Design review of the part built by this model. Coordinates are the model's own, in mm. Face numbers are marked on the shaded views. Give positions to 0.01 mm unless a question says otherwise; leave off trailing zeros. Loops run counter-clockwise (first coordinate to the right, second up) from the corner with the lowest first, then second, coordinate; pieces in that order, holes last. Notation, with made-up numbers: M 34.5,-7.5 L 41.5,-7.5 A12 cw 41.5,5.5 Z; hole C -38.75,-8 d1. An arc over 180 degrees is marked long. Use a Markdown table: item, result. Add a question column.
(1) Insertion check: pin 1 Ø17 at (x, y) = (48.87, 80.04) entering from +Z; pin 2 Ø5 at (x, y) = (-173, -226) entering from +Z; pin 3 Ø5 at (x, y) = (-157.5, -162) entering from +Z; pin 4 Ø5.5 at (y, z) = (89, 3.5) entering from +X. Each pin has a flat end and moves straight along its axis. Give the tip position at first contact, or say it passes through.
(2) Add section D-D, the plane x = -145.5. Give the boundary of the cut face in (y, z).
(3) Add section B-B, the plane x = -110.5. Give the boundary of the cut face in (y, z).
(4) For probe 1 along Y at (x, z) = (-95, 8); probe 2 along X at (y, z) = (-222, 8); probe 3 along Y at (x, z) = (-66, 3.25), list the stretches that pass through material, from the lowest coordinate up.
(5) Add section A-A, the plane y = -22. Give the boundary of the cut face in (x, z).
(6) Add section C-C, the plane y = -169. Give the boundary of the cut face in (x, z), then the cut area to 3 significant figures.
(7) Draft analysis for pull direction X (two halves, no side actions). For the marked faces 1 and 2, state which applies: pulls with the +X half, pulls with the -X half, needs draft (parallel to the pull), parting line crosses it, or undercut.
```python
from build123d import *

# Parameters (mm, degrees)
MODEL_R                 = 10.75
MODEL_R_2               = 1.75
MODEL_R_3               = 5.25
MODEL_R_4               = 1.65
SALIENTE_EXTRUIR1_DEPTH = 10
CORTAR_EXTRUIR1_DEPTH   = 5
CORTAR_EXTRUIR2_DEPTH   = 3
CROQUIS3_R              = 5.1
CORTAR_EXTRUIR3_DEPTH   = 4
CORTAR_EXTRUIR4_REACH   = 307.225
CROQUIS4_R              = 50
CORTAR_EXTRUIR5_REACH   = 307.141


with BuildPart() as part:
    # Model → Saliente-Extruir1 (new body)
    with BuildSketch(Plane.XY):
        with BuildLine():
            Line((-155.7898, 91.0382), (-155.7898, 58.205145042))
            ThreePointArc((-155.7898, 58.205145042), (-156.112526651, 56.437911606), (-157.039045607, 54.898811501))
            Line((-157.039045607, 54.898811501), (-188.380554393, 19.344533541))
            ThreePointArc((-188.380554393, 19.344533541), (-189.307073349, 17.805433436), (-189.6298, 16.0382))
            Line((-189.6298, 16.0382), (-189.6298, -233.9618))
            ThreePointArc((-189.6298, -233.9618), (-188.165333906, -237.497333906), (-184.6298, -238.9618))
            Line((-184.6298, -238.9618), (92.3702, -238.9618))
            ThreePointArc((92.3702, -238.9618), (95.905733906, -237.497333906), (97.3702, -233.9618))
            Line((97.3702, -233.9618), (97.3702, 16.0382))
            ThreePointArc((97.3702, 16.0382), (97.047473349, 17.805433436), (96.120954393, 19.344533541))
            Line((96.120954393, 19.344533541), (64.779445607, 54.898811501))
            ThreePointArc((64.779445607, 54.898811501), (63.852926651, 56.437911606), (63.5302, 58.205145042))
            Line((63.5302, 58.205145042), (63.5302, 91.0382))
            ThreePointArc((63.5302, 91.0382), (62.065733906, 94.573733906), (58.5302, 96.0382))
            Line((58.5302, 96.0382), (-150.7898, 96.0382))
            ThreePointArc((-150.7898, 96.0382), (-154.325333906, 94.573733906), (-155.7898, 91.0382))
        make_face()
        with Locations((48.8702, 80.0382)):
            Circle(MODEL_R, mode=Mode.SUBTRACT)
        with Locations((37.5552, 68.7232)):
            Circle(MODEL_R_2, mode=Mode.SUBTRACT)
        with Locations((60.1852, 68.7232)):
            Circle(MODEL_R_2, mode=Mode.SUBTRACT)
        with Locations((60.1852, 91.3532)):
            Circle(MODEL_R_2, mode=Mode.SUBTRACT)
        with Locations((37.5552, 91.3532)):
            Circle(MODEL_R_2, mode=Mode.SUBTRACT)
        with Locations(Location((-129.8148, 91.3532, 0), (0, 0, 180))):
            Circle(MODEL_R_2, mode=Mode.SUBTRACT)
        with Locations(Location((-152.4448, 91.3532, 0), (0, 0, 180))):
            Circle(MODEL_R_2, mode=Mode.SUBTRACT)
        with Locations(Location((-152.4448, 68.7232, 0), (0, 0, 180))):
            Circle(MODEL_R_2, mode=Mode.SUBTRACT)
        with Locations(Location((-129.8148, 68.7232, 0), (0, 0, 180))):
            Circle(MODEL_R_2, mode=Mode.SUBTRACT)
        with Locations(Location((-141.1298, 80.0382, 0), (0, 0, 180))):
            Circle(MODEL_R, mode=Mode.SUBTRACT)
        with Locations((-46.1298, 80.0382)):
            Circle(MODEL_R_3, mode=Mode.SUBTRACT)
        with Locations((-51.8798, 85.7882)):
            Circle(MODEL_R_4, mode=Mode.SUBTRACT)
        with Locations((-40.3798, 85.7882)):
            Circle(MODEL_R_4, mode=Mode.SUBTRACT)
        with Locations((-40.3798, 74.2882)):
            Circle(MODEL_R_4, mode=Mode.SUBTRACT)
        with Locations((-51.8798, 74.2882)):
            Circle(MODEL_R_4, mode=Mode.SUBTRACT)
    extrude(amount=SALIENTE_EXTRUIR1_DEPTH)

    # Croquis1 → Cortar-Extruir1 (cut)
    with BuildSketch(Plane.XY.offset(10)):
        with BuildLine():
            Line((-167.1298, -229.4618), (-167.1298, 11.5382))
            ThreePointArc((-167.1298, 11.5382), (-166.983353391, 11.891753391), (-166.6298, 12.0382))
            Line((-166.6298, 12.0382), (74.3702, 12.0382))
            ThreePointArc((74.3702, 12.0382), (74.723753391, 11.891753391), (74.8702, 11.5382))
            Line((74.8702, 11.5382), (74.8702, -229.4618))
            ThreePointArc((74.8702, -229.4618), (74.723753391, -229.815353391), (74.3702, -229.9618))
            Line((74.3702, -229.9618), (-166.6298, -229.9618))
            ThreePointArc((-166.6298, -229.9618), (-166.983353391, -229.815353391), (-167.1298, -229.4618))
        make_face()
    extrude(amount=-CORTAR_EXTRUIR1_DEPTH, mode=Mode.SUBTRACT)

    # Croquis2 → Cortar-Extruir2 (cut)
    with BuildSketch(Plane.XY.offset(10)):
        with BuildLine():
            Line((-182.1298, -233.9618), (-182.1298, 16.0382))
            ThreePointArc((-182.1298, 16.0382), (-181.836906781, 16.745306781), (-181.1298, 17.0382))
            Line((-181.1298, 17.0382), (88.8702, 17.0382))
            ThreePointArc((88.8702, 17.0382), (89.577306781, 16.745306781), (89.8702, 16.0382))
            Line((89.8702, 16.0382), (89.8702, -233.9618))
            ThreePointArc((89.8702, -233.9618), (89.577306781, -234.668906781), (88.8702, -234.9618))
            Line((88.8702, -234.9618), (-181.1298, -234.9618))
            ThreePointArc((-181.1298, -234.9618), (-181.836906781, -234.668906781), (-182.1298, -233.9618))
        make_face()
    extrude(amount=-CORTAR_EXTRUIR2_DEPTH, mode=Mode.SUBTRACT)

    # Croquis3 → Cortar-Extruir3 (cut)
    with BuildSketch(Plane.XY.offset(7)):
        with Locations((-174.6298, -227.4618)):
            Circle(CROQUIS3_R)
        with Locations(Location((82.3702, -227.4618, 0), (0, 0, 180))):
            Circle(CROQUIS3_R)
        with Locations(Location((-174.6298, 9.5382, 0), (0, 0, 180))):
            Circle(CROQUIS3_R)
        with Locations((82.3702, 9.5382)):
            Circle(CROQUIS3_R)
    extrude(amount=-CORTAR_EXTRUIR3_DEPTH, mode=Mode.SUBTRACT)

    # Croquis4 → Cortar-Extruir4 (cut, up to next)
    with BuildSketch(Plane(origin=(0, 0, 0), x_dir=(-1, 0, 0), z_dir=(0, 0, -1)), mode=Mode.PRIVATE) as cortar_extruir4_sk1:
        with Locations((46.1298, -281.9618)):
            Circle(CROQUIS4_R)
    cortar_extruir4_tool1 = extrude(cortar_extruir4_sk1.sketch, amount=-CORTAR_EXTRUIR4_REACH, mode=Mode.PRIVATE) & part.part
    add(cortar_extruir4_tool1.solids().sort_by_distance((-46.1298, -281.9618, 0))[0], mode=Mode.SUBTRACT)

    # Croquis5 → Cortar-Extruir5 (cut, up to next)
    with BuildSketch(Plane.XY.offset(7), mode=Mode.PRIVATE) as cortar_extruir5_sk1:
        with BuildLine():
            Line((-71.1298, -27.9618), (-71.1298, 12.0382))
            Line((-71.1298, 12.0382), (-48.1298, 12.0382))
            Line((-48.1298, 12.0382), (-48.1298, 33.205145042))
            ThreePointArc((-48.1298, 33.205145042), (-54.866344033, 49.468601009), (-71.1298, 56.205145042))
            Line((-71.1298, 56.205145042), (-75.9598, 56.205145042))
            ThreePointArc((-75.9598, 56.205145042), (-95.051683092, 64.11326195), (-102.9598, 83.205145042))
            Line((-102.9598, 83.205145042), (-102.9598, 96.0382))
            Line((-102.9598, 96.0382), (-98.9598, 96.0382))
            Line((-98.9598, 96.0382), (-98.9598, 83.205145042))
            ThreePointArc((-98.9598, 83.205145042), (-92.223255967, 66.941689074), (-75.9598, 60.205145042))
            Line((-75.9598, 60.205145042), (-71.1298, 60.205145042))
            ThreePointArc((-71.1298, 60.205145042), (-52.037916908, 52.297028134), (-44.1298, 33.205145042))
            Line((-44.1298, 33.205145042), (-44.1298, 12.0382))
            Line((-44.1298, 12.0382), (-21.1298, 12.0382))
            Line((-21.1298, 12.0382), (-21.1298, -27.9618))
            Line((-21.1298, -27.9618), (-71.1298, -27.9618))
        make_face()
    cortar_extruir5_tool1 = extrude(cortar_extruir5_sk1.sketch, amount=-CORTAR_EXTRUIR5_REACH, mode=Mode.PRIVATE) & part.part
    add(cortar_extruir5_tool1.solids().sort_by_distance((-50.971663, 4.050415, 7))[0], mode=Mode.SUBTRACT)


solid = part.part
```
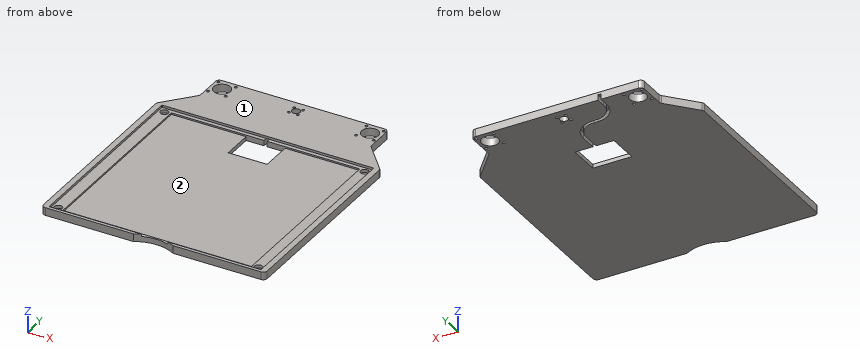
Established:
| question | item | result |
|---|---|---|
| 1 | pin 1 | through |
| 1 | pin 2 | z = 3 |
| 1 | pin 3 | z = 5 |
| 1 | pin 4 | x = 63.53 |
| 2 | outline | M -238.96,0 L 70.22,0 L 70.22,10 L 17.04,10 L 17.04,7 L 12.04,7 L 12.04,5 L -229.96,5 L -229.96,7 L -234.96,7 L -234.96,10 L -238.96,10 Z; M 89.86,0 L 96.04,0 L 96.04,10 L 89.86,10 Z |
| 3 | outline | M -238.96,0 L 96.04,0 L 96.04,10 L 17.04,10 L 17.04,7 L 12.04,7 L 12.04,5 L -229.96,5 L -229.96,7 L -234.96,7 L -234.96,10 L -238.96,10 Z |
| 4 | probe 1 | -238.96 to -234.96, 17.04 to 96.04 |
| 4 | probe 2 | -189.63 to -182.13, 89.87 to 97.37 |
| 4 | probe 3 | -236.08 to -27.96, 12.04 to 55.63, 59.71 to 96.04 |
| 5 | outline | M -189.63,0 L -71.13,0 L -71.13,5 L -167.13,5 L -167.13,7 L -182.13,7 L -182.13,10 L -189.63,10 Z; M -21.13,0 L 97.37,0 L 97.37,10 L 89.87,10 L 89.87,7 L 74.87,7 L 74.87,5 L -21.13,5 Z |
| 6 | outline | M -189.63,0 L 97.37,0 L 97.37,10 L 89.87,10 L 89.87,7 L 74.87,7 L 74.87,5 L -167.13,5 L -167.13,7 L -182.13,7 L -182.13,10 L -189.63,10 Z |
| 6 | area | 1,570 mm^2 |
| 7 | face 1 | needs draft |
| 7 | face 2 | undercut |
